Build history of the part. All positions in model axes, mm. A direction names the side the tool comes from. Round coordinates to 2 decimals unless told otherwise and drop trailing zeros. Loops run counter-clockwise (first coordinate to the right, second up) from the corner with the lowest first, then second, coordinate; pieces in that order, holes last. Notation, with made-up numbers: (12, 12.5) - (53, 12.5) arc R17 cw to (53, 42.5) - close; hole circle Ø4 at (89.5, 8.5). An arc over 180 degrees is marked (long way). Put each result on its own line as item: value. Start each with the question number.
from build123d import *

# Parameters (mm, degrees)
F0_R      = 350
F1_DEPTH  = 25
F3_DEPTH  = 25
F4_R      = 335
F5_DEPTH  = 15
F6_R      = 2
F6_R_2    = 1.5
F7_DEPTH  = 25
F8_R      = 3.55
F9_DEPTH  = 4
F11_DEPTH = 25
F12_R     = 1.778
F13_DEPTH = 25


with BuildPart() as f1:
    # F0 (on Top) → F1 (new body)
    with BuildSketch(Plane.XY):
        Circle(F0_R)
    extrude(amount=F1_DEPTH)

    # F2 (on face) → F3 (cut)
    with BuildSketch(Plane.XY.offset(25)):
        with BuildLine():
            Line((50, 335), (0, 335))
            Line((0, 335), (0, 265))
            Line((0, 265), (50, 265))
            ThreePointArc((50, 265), (57.071068, 267.928932), (60, 275))
            Line((60, 275), (60, 325))
            ThreePointArc((60, 325), (57.071068, 332.071068), (50, 335))
        make_face()
        with BuildLine():
            Line((265, 50), (265, 0))
            Line((265, 0), (335, 0))
            Line((335, 0), (335, 50))
            ThreePointArc((335, 50), (332.071068, 57.071068), (325, 60))
            Line((325, 60), (275, 60))
            ThreePointArc((275, 60), (267.928932, 57.071068), (265, 50))
        make_face()
        with BuildLine():
            Line((335, 0), (265, 0))
            Line((265, 0), (265, -50))
            ThreePointArc((265, -50), (267.928932, -57.071068), (275, -60))
            Line((275, -60), (325, -60))
            ThreePointArc((325, -60), (332.071068, -57.071068), (335, -50))
            Line((335, -50), (335, 0))
        make_face()
        with BuildLine():
            Line((50, -265), (0, -265))
            Line((0, -265), (0, -335))
            Line((0, -335), (50, -335))
            ThreePointArc((50, -335), (57.071068, -332.071068), (60, -325))
            Line((60, -325), (60, -275))
            ThreePointArc((60, -275), (57.071068, -267.928932), (50, -265))
        make_face()
        with BuildLine():
            Line((0, -335), (0, -265))
            Line((0, -265), (-50, -265))
            ThreePointArc((-50, -265), (-57.071068, -267.928932), (-60, -275))
            Line((-60, -275), (-60, -325))
            ThreePointArc((-60, -325), (-57.071068, -332.071068), (-50, -335))
            Line((-50, -335), (0, -335))
        make_face()
        with BuildLine():
            Line((-265, -50), (-265, 0))
            Line((-265, 0), (-335, 0))
            Line((-335, 0), (-335, -50))
            ThreePointArc((-335, -50), (-332.071068, -57.071068), (-325, -60))
            Line((-325, -60), (-275, -60))
            ThreePointArc((-275, -60), (-267.928932, -57.071068), (-265, -50))
        make_face()
        with BuildLine():
            Line((-335, 0), (-265, 0))
            Line((-265, 0), (-265, 50))
            ThreePointArc((-265, 50), (-267.928932, 57.071068), (-275, 60))
            Line((-275, 60), (-325, 60))
            ThreePointArc((-325, 60), (-332.071068, 57.071068), (-335, 50))
            Line((-335, 50), (-335, 0))
        make_face()
        with BuildLine():
            Line((0, 265), (0, 335))
            Line((0, 335), (-50, 335))
            ThreePointArc((-50, 335), (-57.071068, 332.071068), (-60, 325))
            Line((-60, 325), (-60, 275))
            ThreePointArc((-60, 275), (-57.071068, 267.928932), (-50, 265))
            Line((-50, 265), (0, 265))
        make_face()
    extrude(amount=-F3_DEPTH, mode=Mode.SUBTRACT)

    # F4 (on face) → F5 (cut)
    with BuildSketch(Plane.XY.offset(25)):
        Circle(F4_R)
    extrude(amount=-F5_DEPTH, mode=Mode.SUBTRACT)

    # F6 (on face) → F7 (cut)
    with BuildSketch(Plane.XY.offset(10)):
        with Locations((-233.162066, 23.69)):
            Circle(F6_R)
        with BuildLine():
            Line((-214.542066, 23.69), (-210.542066, 23.69))
            ThreePointArc((-210.542066, 23.69), (-212.542066, 25.69), (-214.542066, 23.69))
        make_face()
        with BuildLine():
            ThreePointArc((-214.542066, 23.69), (-212.542066, 21.69), (-210.542066, 23.69))
            Line((-210.542066, 23.69), (-214.542066, 23.69))
        make_face()
        with Locations((-233.162066, -23.69)):
            Circle(F6_R)
        with BuildLine():
            Line((-214.542066, -23.69), (-210.542066, -23.69))
            ThreePointArc((-210.542066, -23.69), (-212.542066, -21.69), (-214.542066, -23.69))
        make_face()
        with BuildLine():
            ThreePointArc((-214.542066, -23.69), (-212.542066, -25.69), (-210.542066, -23.69))
            Line((-210.542066, -23.69), (-214.542066, -23.69))
        make_face()
        with Locations((-23.69, -233.162066)):
            Circle(F6_R)
        with Locations((-23.69, -212.542066)):
            Circle(F6_R)
        with Locations((23.69, -212.542066)):
            Circle(F6_R)
        with Locations((23.69, -233.162066)):
            Circle(F6_R)
        with Locations((233.162066, -23.69)):
            Circle(F6_R)
        with Locations((212.542066, -23.69)):
            Circle(F6_R)
        with Locations((212.542066, 23.69)):
            Circle(F6_R)
        with Locations((233.162066, 23.69)):
            Circle(F6_R)
        with Locations((23.69, 233.162066)):
            Circle(F6_R)
        with Locations((23.69, 212.542066)):
            Circle(F6_R)
        with Locations((-23.69, 212.542066)):
            Circle(F6_R)
        with Locations((-23.69, 233.162066)):
            Circle(F6_R)
        with Locations((-173.937469, 8.69)):
            Circle(F6_R_2)
        with Locations((-173.937469, -8.69)):
            Circle(F6_R_2)
        with Locations((-155, 8.69)):
            Circle(F6_R_2)
        with Locations((-8.69, -173.937469)):
            Circle(F6_R_2)
        with Locations((-8.69, -155)):
            Circle(F6_R_2)
        with Locations((8.69, -173.937469)):
            Circle(F6_R_2)
        with Locations((173.937469, -8.69)):
            Circle(F6_R_2)
        with Locations((155, -8.69)):
            Circle(F6_R_2)
        with Locations((173.937469, 8.69)):
            Circle(F6_R_2)
        with Locations((8.69, 173.937469)):
            Circle(F6_R_2)
        with Locations((8.69, 155)):
            Circle(F6_R_2)
        with Locations((-8.69, 173.937469)):
            Circle(F6_R_2)
        with Locations((-155, -8.69)):
            Circle(F6_R_2)
        with Locations((8.69, -155)):
            Circle(F6_R_2)
        with Locations((155, 8.69)):
            Circle(F6_R_2)
        with Locations((-8.69, 155)):
            Circle(F6_R_2)
    extrude(amount=-F7_DEPTH, mode=Mode.SUBTRACT)

    # F8 (on face) → F9 (cut)
    with BuildSketch(Plane.XY.offset(10)):
        with Locations((23.69, 233.162066)):
            Circle(F8_R)
        with Locations((23.69, 212.542066)):
            Circle(F8_R)
        with Locations((-23.69, 233.162066)):
            Circle(F8_R)
        with Locations((-23.69, 212.542066)):
            Circle(F8_R)
        with Locations((-212.542066, 23.69)):
            Circle(F8_R)
        with Locations((-233.162066, 23.69)):
            Circle(F8_R)
        with Locations((-233.162066, -23.69)):
            Circle(F8_R)
        with Locations((-212.542066, -23.69)):
            Circle(F8_R)
        with Locations((-23.69, -212.542066)):
            Circle(F8_R)
        with Locations((-23.69, -233.162066)):
            Circle(F8_R)
        with Locations((23.69, -233.162066)):
            Circle(F8_R)
        with Locations((23.69, -212.542066)):
            Circle(F8_R)
        with Locations((212.542066, -23.69)):
            Circle(F8_R)
        with Locations((233.162066, -23.69)):
            Circle(F8_R)
        with Locations((233.162066, 23.69)):
            Circle(F8_R)
        with Locations((212.542066, 23.69)):
            Circle(F8_R)
    extrude(amount=-F9_DEPTH, mode=Mode.SUBTRACT)

    # F10 (on face) → F11 (cut)
    with BuildSketch(Plane.XY.offset(10)):
        with BuildLine():
            Line((-47.5, 10), (-47.5, 0))
            Line((-47.5, 0), (-32.5, 0))
            Line((-32.5, 0), (-32.5, 10))
            ThreePointArc((-32.5, 10), (-33.964466, 13.535534), (-37.5, 15))
            Line((-37.5, 15), (-42.5, 15))
            ThreePointArc((-42.5, 15), (-46.035534, 13.535534), (-47.5, 10))
        make_face()
        with BuildLine():
            Line((-32.5, 0), (-47.5, 0))
            Line((-47.5, 0), (-47.5, -10))
            ThreePointArc((-47.5, -10), (-46.035534, -13.535534), (-42.5, -15))
            Line((-42.5, -15), (-37.5, -15))
            ThreePointArc((-37.5, -15), (-33.964466, -13.535534), (-32.5, -10))
            Line((-32.5, -10), (-32.5, 0))
        make_face()
        with BuildLine():
            Line((32.5, 10), (32.5, 0))
            Line((32.5, 0), (47.5, 0))
            Line((47.5, 0), (47.5, 10))
            ThreePointArc((47.5, 10), (46.035534, 13.535534), (42.5, 15))
            Line((42.5, 15), (37.5, 15))
            ThreePointArc((37.5, 15), (33.964466, 13.535534), (32.5, 10))
        make_face()
        with BuildLine():
            Line((47.5, 0), (32.5, 0))
            Line((32.5, 0), (32.5, -10))
            ThreePointArc((32.5, -10), (33.964466, -13.535534), (37.5, -15))
            Line((37.5, -15), (42.5, -15))
            ThreePointArc((42.5, -15), (46.035534, -13.535534), (47.5, -10))
            Line((47.5, -10), (47.5, 0))
        make_face()
    extrude(amount=-F11_DEPTH, mode=Mode.SUBTRACT)

    # F12 (on face) → F13 (cut)
    with BuildSketch(Plane.XY.offset(10)):
        with Locations((-169.697342, 211.186125)):
            Circle(F12_R)
        with Locations((-211.186125, 169.697342)):
            Circle(F12_R)
        with Locations((-180.315964, 138.827181)):
            Circle(F12_R)
        with Locations((-138.827181, 180.315964)):
            Circle(F12_R)
        with Locations((211.186125, -169.697342)):
            Circle(F12_R)
        with Locations((180.315964, -138.827181)):
            Circle(F12_R)
        with Locations((138.827181, -180.315964)):
            Circle(F12_R)
        with Locations((169.697342, -211.186125)):
            Circle(F12_R)
    extrude(amount=-F13_DEPTH, mode=Mode.SUBTRACT)


solid = f1.part
1) Slice it at A-A, the plane x = 253.5. Write the cut outline in (y, z), and give its area (3 significant figures).
2) Which spindle directions (+Z, -Z, +X, -X, +Y, -Y) get a long thin tool onto all of the face, cutting with end or side? Do faces 1 (the face through (-335, 1, 13)), 2 (the face through (284, -180, 25)), 3 (the face through (234.852, -238.892, 17.605)). Say none if no direction does.
3) Pull direction X, two halves, no side cores. Call faces 4 (the face through (-257.96, 236.55, 12.32)), 5 (the face through (-5, 5, 0)), 6 (the face through (-234.852, 238.892, 17.605)): pulls with the +X half, pulls with the -X half, needs draft (parallel to the pull), parting line crosses it, or undercut.
4) Slice it at B-B, the plane y = -85. Write the cut outline in (x, z).
5) Drop flat-ended pins along their axis: pin 1 Ø5.5 at (x, y) = (22, 213) entering from +Z; pin 2 Ø5.5 at (x, y) = (212.54, -23.69) entering from +Z; pin 3 Ø1 at (y, z) = (-255.5, 10.5) entering from -X; pin 4 Ø3.5 at (x, y) = (-23.69, -212.54) entering from +Z. Give the stop position or say it passes through.
6) Drill centre lines: line 1 (Y direction, x = -20.5, z = 2.75); line 2 (X direction, y = 40.5, z = 6.5); line 3 (Y direction, x = -55, z = 4.75). Where is each one in solid material? Low to high. Write a range as [from, to].
Taken from the geometry:
1. outline: (-241.32, 0) - (241.32, 0) - (241.32, 25) - (219, 25) - (219, 10) - (-219, 10) - (-219, 25) - (-241.32, 25) - close
1. area: 5,500 mm2
2. face 1: +Z, -Z
2. face 2: +Z, +X, -X, +Y, -Y
2. face 3: +Z
3. face 4: parting line crosses it
3. face 5: needs draft
3. face 6: undercut
4. outline: (-339.52, 0) - (339.52, 0) - (339.52, 25) - (324.04, 25) - (324.04, 10) - (-324.04, 10) - (-324.04, 25) - (-339.52, 25) - close
5. pin 1: stops at z = 10
5. pin 2: stops at z = 6
5. pin 3: stops at x = -239.74
5. pin 4: passes through
6. line 1: y = [-349.4, -335], [-265, 265], [335, 349.4]
6. line 2: x = [-347.65, -335], [-265, 265], [335, 347.65]
6. line 3: y = [-345.65, -333.66], [-266.34, 266.34], [333.66, 345.65]
